from build123d import *

# Parameters (mm, degrees)
SKETCH1_W           = 36
SKETCH1_H           = 20
BOSS_EXTRUDE1_DEPTH = 2
SKETCH2_W           = 36
SKETCH2_H           = 2
BOSS_EXTRUDE2_DEPTH = 36
CUT_EXTRUDE1_REACH  = 48.562
SKETCH3_R           = 1.5
CUT_EXTRUDE3_REACH  = 43.473
SKETCH4_R           = 1.5
FILLET1_R           = 1


with BuildPart() as part:
    # Sketch1 → Boss-Extrude1 (new body)
    with BuildSketch(Plane(origin=(0, 0, 0), x_dir=(1, 0, 0), z_dir=(0, 1, 0))):
        Rectangle(SKETCH1_W, SKETCH1_H)
    extrude(amount=BOSS_EXTRUDE1_DEPTH)

    # Sketch2 → Boss-Extrude2 (add)
    with BuildSketch(Plane(origin=(0, 2, 0), x_dir=(1, 0, 0), z_dir=(0, 1, 0))):
        with Locations((0, 9)):
            Rectangle(SKETCH2_W, SKETCH2_H)
    extrude(amount=BOSS_EXTRUDE2_DEPTH)

    # Sketch3 → Cut-Extrude1 (cut, up to next)
    with BuildSketch(Plane(origin=(0, 0, -10), x_dir=(-1, 0, 0), z_dir=(0, 0, -1)), mode=Mode.PRIVATE) as cut_extrude1_sk1:
        with Locations((-14.4, 33.4)):
            Circle(SKETCH3_R)
    cut_extrude1_tool1 = extrude(cut_extrude1_sk1.sketch, amount=-CUT_EXTRUDE1_REACH, mode=Mode.PRIVATE) & part.part
    # Sketch3 → Cut-Extrude1 (cut, up to next)
    with BuildSketch(Plane(origin=(0, 0, -10), x_dir=(-1, 0, 0), z_dir=(0, 0, -1)), mode=Mode.PRIVATE) as cut_extrude1_sk2:
        with Locations((14.4, 33.4)):
            Circle(SKETCH3_R)
    cut_extrude1_tool2 = extrude(cut_extrude1_sk2.sketch, amount=-CUT_EXTRUDE1_REACH, mode=Mode.PRIVATE) & part.part
    # Sketch3 → Cut-Extrude1 (cut, up to next)
    with BuildSketch(Plane(origin=(0, 0, -10), x_dir=(-1, 0, 0), z_dir=(0, 0, -1)), mode=Mode.PRIVATE) as cut_extrude1_sk3:
        with Locations((14.4, 4.6)):
            Circle(SKETCH3_R)
    cut_extrude1_tool3 = extrude(cut_extrude1_sk3.sketch, amount=-CUT_EXTRUDE1_REACH, mode=Mode.PRIVATE) & part.part
    # Sketch3 → Cut-Extrude1 (cut, up to next)
    with BuildSketch(Plane(origin=(0, 0, -10), x_dir=(-1, 0, 0), z_dir=(0, 0, -1)), mode=Mode.PRIVATE) as cut_extrude1_sk4:
        with Locations((-14.4, 4.6)):
            Circle(SKETCH3_R)
    cut_extrude1_tool4 = extrude(cut_extrude1_sk4.sketch, amount=-CUT_EXTRUDE1_REACH, mode=Mode.PRIVATE) & part.part
    add(cut_extrude1_tool1.solids().sort_by_distance((14.4, 33.4, -10))[0], mode=Mode.SUBTRACT)
    add(cut_extrude1_tool2.solids().sort_by_distance((-14.4, 33.4, -10))[0], mode=Mode.SUBTRACT)
    add(cut_extrude1_tool3.solids().sort_by_distance((-14.4, 4.6, -10))[0], mode=Mode.SUBTRACT)
    add(cut_extrude1_tool4.solids().sort_by_distance((14.4, 4.6, -10))[0], mode=Mode.SUBTRACT)

    # Sketch4 → Cut-Extrude3 (cut, up to next)
    with BuildSketch(Plane(origin=(0, 2, 0), x_dir=(1, 0, 0), z_dir=(0, 1, 0)), mode=Mode.PRIVATE) as cut_extrude3_sk1:
        with Locations(Location((0, -1, 0), (0, 0, 270))):
            Circle(SKETCH4_R)
    cut_extrude3_tool1 = extrude(cut_extrude3_sk1.sketch, amount=-CUT_EXTRUDE3_REACH, mode=Mode.PRIVATE) & part.part
    add(cut_extrude3_tool1.solids().sort_by_distance((0, 2, 1))[0], mode=Mode.SUBTRACT)

    # Fillet1
    fillet1_edges = [part.edges().sort_by_distance(p)[0] for p in [
        (0, 2, 10),
        (-18, 2, 1),
        (0, 2, -8),
        (-18, 20, -8),
        (18, 20, -8),
        (-18, 38, -9),
        (0, 38, -8),
        (18, 38, -9),
        (18, 2, 1),
        (0, 0, -10),
    ]]
    fillet(fillet1_edges, radius=FILLET1_R)


solid = part.part
Here's how the part is built. I have some questions about the finished solid (model axes, mm). A direction names the side the tool comes from. Round coordinates to 2 decimals unless told otherwise and drop trailing zeros. Order: outer loops, then holes, each group sorted by start corner. A loop starts at its lowest first (then second) coordinate and runs counter-clockwise, first axis right, second up. Notation, with made-up numbers: (78.25, -14.75) -> (85.25, -14.75) arc R13 ccw to (85.25, 4.25) -> close; hole circle Ø2 at (-37.75, 41). An arc over 180 degrees is marked (long way). Return JSON: item names as keys, results as strings.
Q1. If we section it at C-C on x = -14.4: List the corners of the cut face in (y, z) for me, plus the area to 3 significant figures.
Filled sheet:
{"outline": "(0, -9) arc R1 ccw to (1, -10) -> (3.1, -10) -> (3.1, -8) -> (3, -8) arc R1 cw to (2, -7) -> (2, 9) arc R1 ccw to (1, 10) -> (0, 10) -> close; (6.1, -10) -> (31.9, -10) -> (31.9, -8) -> (6.1, -8) -> close; (34.9, -10) -> (38, -10) -> (38, -9) arc R1 ccw to (37, -8) -> (34.9, -8) -> close", "area": "99.6 mm^2"}
Q2. If we section it at D-D on y = 7: List the corners of the cut face in (x, z) for me, plus the area to 3 significant figures.
Filled sheet:
{"outline": "(-18, -10) -> (18, -10) -> (18, -9) arc R1 ccw to (17, -8) -> (-17, -8) arc R1 ccw to (-18, -9) -> close", "area": "71.6 mm^2"}
Q3. If we section it at B-B on y = 33.4: List the corners of the cut face in (x, z) for me.
Filled sheet:
{"outline": "(-18, -10) -> (-15.9, -10) -> (-15.9, -8) -> (-17, -8) arc R1 ccw to (-18, -9) -> close; (-12.9, -10) -> (12.9, -10) -> (12.9, -8) -> (-12.9, -8) -> close; (15.9, -10) -> (18, -10) -> (18, -9) arc R1 ccw to (17, -8) -> (15.9, -8) -> close"}
Q4. For pin 1 Ø12 at (x, y) = (-11, 33) entering from +Z; pin 2 Ø12 at (x, z) = (-1, -1) entering from +Y; pin 3 Ø1.8 at (x, y) = (14.4, 4.6) entering from -Z; pin 4 Ø2 at (x, z) = (-13, -7.5) entering from +Y, each with a flat end and sliding along its axis, tell me the tip position at first contact or that it passes through.
Filled sheet:
{"pin 1": "stops at z = -8", "pin 2": "stops at y = 2", "pin 3": "passes through", "pin 4": "stops at y = 37.87"}
Q5. If we mould it in two halves opening along Y, with no side actions, what happens to faces 3 (the cylindrical face through (-0.575, 1.014, 2.386)), 4 (the cylindrical face through (15.9, 4.67, -9.01)), 5 (the cylindrical face through (17.699, 1.715, 1.381))? For each: released by +Y, released by -Y, zero draft, split by the parting line, or undercut.
Filled sheet:
{"face 3": "zero draft", "face 4": "undercut", "face 5": "released by +Y"}
Q6. If we section it at A-A on z = 1: List the corners of the cut face in (x, y) for me.
Filled sheet:
{"outline": "(-18, 0) -> (-1.5, 0) -> (-1.5, 2) -> (-17, 2) arc R1 ccw to (-18, 1) -> close; (1.5, 0) -> (18, 0) -> (18, 1) arc R1 ccw to (17, 2) -> (1.5, 2) -> close"}
Q7. Which directions (+Z, -Z, +X, -X, +Y, -Y) give clear straight access to the entire face, cutting with the end or side of a thin tool? Please do faces 1 (the cylindrical face through (0.252, 0.301, -9.715)), 2 (the cylindrical face through (-17.715, 20.238, -8.301)).
Filled sheet:
{"face 1": "-Z, +X, -X, -Y", "face 2": "+Z, -X, +Y"}
Q8. I need wall thicknesses on line 1 along Y through (x, z) = (-14.4, -9.05); line 2 along X through (y, z) = (0.65, 1); line 3 along Z through (x, y) = (12.5, 12). Which ranges of each line are inside material? Lowest first, please. Write a range as from..to.
Filled sheet:
{"line 1": "y = 0..3.1, 6.1..31.9, 34.9..38", "line 2": "x = -18..-1.5, 1.5..18", "line 3": "z = -10..-8"}
